Autodesk Inventor part; units mm, degrees
ref_plane "YZ Plane" through (0, 0, 0) normal (1, 0, 0) x (0, 1, 0)
ref_plane "XZ Plane" through (0, 0, 0) normal (0, 1, 0) x (-1, 0, 0)
ref_plane "XY Plane" through (0, 0, 0) normal (0, 0, 1) x (1, 0, 0)
sketch "スケッチ1" plane through (0, 0, 0) normal (0, 0, 1) x (1, 0, 0)
  circle A0 centre (0, 0) radius 1.5
  dimension "d0" = 3
extrude "押し出し1" add sketch "スケッチ1" along normal blind 6
sketch "スケッチ2" plane through (0, 0, 6) normal (0, 0, 1) x (1, 0, 0)
  circle A0 centre (0, 0) radius 1.5
  circle A1 centre (0, 0) radius 3
  dimension "d3" = 6
extrude "押し出し2" add sketch "スケッチ2" along normal blind 1.75 contours A0 | A1
thread "ねじ1"
chamfer "面取り1" distance 1.5 angle 45 1 edges at (-3, 0, 6)
sketch "スケッチ4" plane through (0, 0, 0) normal (0, 0, -1) x (-1, 0, 0)
  circle A0 centre (0, 0) radius 1.5
extrude "押し出し4" add sketch "スケッチ4" along normal blind 4
sketch "スケッチ5" plane through (0, 0, -4) normal (0, 0, -1) x (-1, 0, 0)
  circle A0 centre (0, 0) radius 1.5
extrude "押し出し5" cut sketch "スケッチ5" against normal blind 2
sketch "スケッチ6" plane through (0, 0, -2) normal (0, 0, -1) x (-1, 0, 0)
  circle A0 centre (0, 0) radius 1.5
extrude "押し出し6" add sketch "スケッチ6" along normal blind 2.25
properties part number "SB　12mm皿ネジ" material "Steel, Mild"
CAD build for the part. Positions are in the model's coordinates, mm. Round coordinates to 2 decimals unless told otherwise and drop trailing zeros. Order: outer loops, then holes, each group sorted by start corner. A loop starts at its lowest first (then second) coordinate and runs counter-clockwise, first axis right, second up. Notation, with made-up numbers: (38.25, 42) -> (92.25, 42) arc R22 ccw to (92.25, 76) -> close; hole circle Ø7 at (-39, 38.25). An arc over 180 degrees is marked (long way). Write item = value, one per line. Start each with the question number.
(1) Cut at C-C, the plane z = 7.25. List the corners of the cut face in (x, y).
(2) Pin check, flat tips, straight feed: P1, Ø1.5, axis at y = 0, z = 6.5, coming from the -X side; P2, Ø1.5, axis at y = 1.5, z = 2, coming from the +X side; P3, Ø1.5, axis at y = 1.5, z = 0.5, coming from the -X side. Stop position of each tip, or through.
(3) Probe line 1 (X direction, y = 0.05, z = -2.25); line 2 (Z direction, x = 1.5, y = -2); line 3 (Y direction, x = 0.15, z = 2.5). List the from-to ranges inside material, lowest first. Write a range as [from, to].
(4) Cut at D-D, the plane z = -0.75. List the corners of the cut face in (x, y).
Model answer:
q1.outline = circle Ø5.5 at (0, 0)
q2.P1 = -2.75
q2.P2 = 1.3
q2.P3 = -1.3
q3.line_1 = [-1.5, 1.5]
q3.line_2 = [7, 7.75]
q3.line_3 = [-1.49, 1.49]
q4.outline = circle Ø3 at (0, 0)
